Design review of the part built by this model. Coordinates are the model's own, in mm. Face numbers are marked on the shaded views. Give positions to 0.01 mm unless a question says otherwise; leave off trailing zeros. Loops run counter-clockwise (first coordinate to the right, second up) from the corner with the lowest first, then second, coordinate; pieces in that order, holes last. Notation, with made-up numbers: (79, 7.25) -> (120, 7.25) arc R8 ccw to (120, 21.25) -> close; hole circle Ø10 at (3, 35.5). An arc over 180 degrees is marked (long way). Answer in a Markdown table with one row per item. Add a question column.
(1) Consider section B-B on x = 0. Write out the cut boundary in (y, z).
(2) Consider section D-D on y = 55. Write out the cut boundary in (x, z).
(3) Consider section A-A on z = 0. Write out the cut boundary in (x, y), then the cut area to 3 significant figures.
(4) Consider section C-C on y = 25. Write out the cut boundary in (x, z), then the cut area to 3 significant figures.
(5) Draft analysis for pull direction Z (two halves, no side actions). For the marked faces 1, 2 and 3, state which applies: +Z half, -Z half, draft (parallel to the pull), parting line (faces both ways), or undercut.
(6) For pin 1 (10 mm diameter, centred on x = -3, y = 43, fed in from -Z); pin 2 (3 mm diameter, centred on x = 13, z = -4.5, fed in from -Y); pin 3 (5 mm diameter, centred on y = 9, z = 3, fed in from -X); pin 4 (6 mm diameter, centred on y = 32, z = 11, fed in from -X), all flat-tipped, find the tip position at first contact; note any pin that passes through.
(7) For line 1 (X direction, y = 29, z = 0); line 2 (Y direction, x = -25.5, z = 13), list the stretches that pass through material, from the lowest coordinate up.
from build123d import *

# Parameters (mm, degrees)
SKETCH_1_R      = 31
EXTRUDE_1_DEPTH = 40
SKETCH_2_R      = 28.5
EXTRUDE_2_DEPTH = 30
FILLET_1_R      = 10
SHELL_1_T       = -3


with BuildPart() as part:
    # 스케치1 → 보스-돌출1 (new body)
    with BuildSketch(Plane(origin=(0, 0, 0), x_dir=(1, 0, 0), z_dir=(0, 1, 0))):
        with Locations(Location((0, 0, 0), (0, 0, 270))):
            Circle(SKETCH_1_R)
    extrude(amount=EXTRUDE_1_DEPTH)

    # 스케치2 → 보스-돌출2 (add)
    with BuildSketch(Plane(origin=(0, 40, 0), x_dir=(1, 0, 0), z_dir=(0, 1, 0))):
        with Locations(Location((0, 0, 0), (0, 0, 270))):
            Circle(SKETCH_2_R)
    extrude(amount=EXTRUDE_2_DEPTH)

    # 필렛1
    fillet_1_edges = [part.edges().sort_by_distance(p)[0] for p in [
        (0, 70, -28.5),
    ]]
    fillet(fillet_1_edges, radius=FILLET_1_R)

    # 쉘1
    shell_1_openings = [part.faces().sort_by_distance(p)[0] for p in [
        (0, 0, 0),
    ]]
    offset(amount=SHELL_1_T, openings=shell_1_openings, kind=Kind.INTERSECTION)


solid = part.part
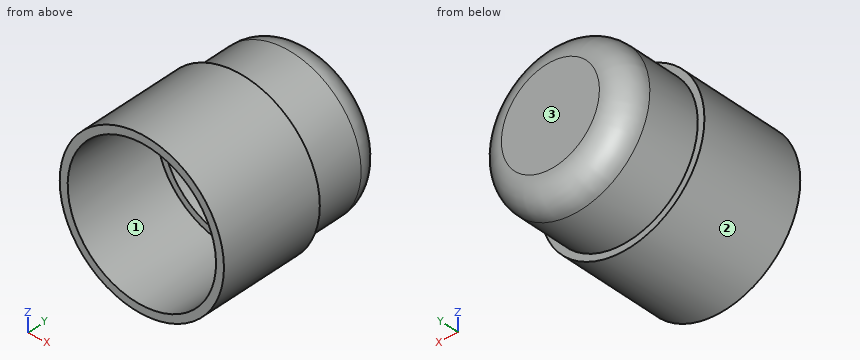
Values follow:
| question | item | result |
|---|---|---|
| 1 | outline | (0, -31) -> (40, -31) -> (40, -28.5) -> (60, -28.5) arc R10 ccw to (70, -18.5) -> (70, 18.5) arc R10 ccw to (60, 28.5) -> (40, 28.5) -> (40, 31) -> (0, 31) -> (0, 28) -> (37, 28) -> (37, 25.5) -> (60, 25.5) arc R7 cw to (67, 18.5) -> (67, -18.5) arc R7 cw to (60, -25.5) -> (37, -25.5) -> (37, -28) -> (0, -28) -> close |
| 2 | outline | circle Ø57 at (0, 0); hole circle Ø51 at (0, 0) |
| 3 | outline | (-31, 0) -> (-28, 0) -> (-28, 37) -> (-25.5, 37) -> (-25.5, 60) arc R7 cw to (-18.5, 67) -> (18.5, 67) arc R7 cw to (25.5, 60) -> (25.5, 37) -> (28, 37) -> (28, 0) -> (31, 0) -> (31, 40) -> (28.5, 40) -> (28.5, 60) arc R10 ccw to (18.5, 70) -> (-18.5, 70) arc R10 ccw to (-28.5, 60) -> (-28.5, 40) -> (-31, 40) -> close |
| 3 | area | 566 mm2 |
| 4 | outline | circle Ø62 at (0, 0); hole circle Ø56 at (0, 0) |
| 4 | area | 556 mm2 |
| 5 | face 1 | undercut |
| 5 | face 2 | parting line |
| 5 | face 3 | draft |
| 6 | pin 1 | z = -31 |
| 6 | pin 2 | y = 67 |
| 6 | pin 3 | x = -31 |
| 6 | pin 4 | x = -29.95 |
| 7 | line 1 | -31 to -28, 28 to 31 |
| 7 | line 2 | 0 to 40 |
